Geometry: final body of the model. Coordinates: model frame, mm. Face numbers are marked on the shaded views. A direction names the side the tool comes from. Give positions to 0.01 mm unless a question says otherwise; leave off trailing zeros. Write each loop counter-clockwise with the first axis right and the second up, starting at its lowest first coordinate (ties: lowest second). Pieces come first, ordered by that corner, then holes.
```python
from build123d import *

# Parameters (mm, degrees)
SKETCH_1_W           = 112
SKETCH_1_H           = 110
EXTRUDE_1_DEPTH      = 126
FILLET_1_R           = 55
SKETCH_9_R           = 42.5
CUT_EXTRUDE_5_DEPTH  = 104
SKETCH_10_R          = 42.5
CUT_EXTRUDE_6_DEPTH  = 57
CUT_EXTRUDE_START    = -50
SKETCH_11_R          = 42.5
CUT_EXTRUDE_7_DEPTH  = 50
CHAMFER_1_SIZE       = 55
CHAMFER_1_SIZE2      = 5
CHAMFER_2_SIZE       = 5
CHAMFER_2_SIZE2      = 55
SKETCH_14_W          = 143.089430894
SKETCH_14_H          = 9
CUT_EXTRUDE_8_DEPTH  = 202.295802241
CHAMFER_5_SIZE       = 4
CHAMFER_6_SIZE       = 4
SKETCH_18_R          = 5
CUT_EXTRUDE_9_DEPTH  = 21
SKETCH_19_R          = 45
CUT_EXTRUDE_10_DEPTH = 11
CUT_EXTRUDE_START_2  = -11
SKETCH_20_R          = 45
CUT_EXTRUDE_11_DEPTH = 11
CHAMFER_7_SIZE       = 4
SKETCH_17_R          = 47.5
SKETCH_17_R_2        = 42.5
CUT_EXTRUDE_12_DEPTH = 2
CHAMFER_8_SIZE       = 1
SKETCH_21_R          = 5
CUT_EXTRUDE_13_DEPTH = 10
SKETCH_22_R          = 2
CUT_EXTRUDE_14_DEPTH = 10


# Some blends are built 0.0001 mm under size
with BuildPart() as part:
    # 草图1 → 拉伸1 (new body)
    with BuildSketch(Plane.XY):
        with Locations((56, -55)):
            Rectangle(SKETCH_1_W, SKETCH_1_H)
    extrude(amount=EXTRUDE_1_DEPTH)

    # 圆角1
    fillet_1_edges = [part.edges().sort_by_distance(p)[0] for p in [
        (112, -110, 63),
        (112, 0, 63),
    ]]
    fillet(fillet_1_edges, radius=FILLET_1_R - 0.0001)  # a hair under: the kernel refuses the full size

    # 草图9 → 切除-拉伸5 (cut)
    with BuildSketch(Plane.XY.offset(126)):
        with Locations((57, -55)):
            Circle(SKETCH_9_R)
    extrude(amount=-CUT_EXTRUDE_5_DEPTH, mode=Mode.SUBTRACT)

    # 草图10 → 切除-拉伸6 (cut)
    with BuildSketch(Plane.ZY):
        with Locations(Location((63, -55, 0), (0, 0, 270))):
            Circle(SKETCH_10_R)
    extrude(amount=-CUT_EXTRUDE_6_DEPTH, mode=Mode.SUBTRACT)

    # 草图11 → 切除-拉伸7 (cut)
    with BuildSketch(Plane(origin=(0, 0, 0), x_dir=(-1, 0, 0), z_dir=(0, 0, -1)).offset(CUT_EXTRUDE_START)):
        with Locations(Location((-57, -55, 0), (0, 0, 180))):
            Circle(SKETCH_11_R)
    extrude(amount=CUT_EXTRUDE_7_DEPTH, mode=Mode.SUBTRACT)

    # 倒角1
    chamfer_1_edges = [part.edges().sort_by_distance(p)[0] for p in [
        (0, 0, 63),
    ]]
    chamfer_1_side = [part.faces().sort_by_distance(p)[0] for p in [
        (28.50005, 0, 63),
    ]]
    chamfer(chamfer_1_edges, length=CHAMFER_1_SIZE, length2=CHAMFER_1_SIZE2, reference=chamfer_1_side[0])

    # 倒角2
    chamfer_2_edges = [part.edges().sort_by_distance(p)[0] for p in [
        (0, -110, 63),
    ]]
    chamfer_2_side = [part.faces().sort_by_distance(p)[0] for p in [
        (0, -57.5, 1.640152432),
    ]]
    chamfer(chamfer_2_edges, length=CHAMFER_2_SIZE, length2=CHAMFER_2_SIZE2, reference=chamfer_2_side[0])

    # 草图14 → 切除-拉伸8 (cut, through all)
    with BuildSketch(Plane(origin=(0, 0, 0), x_dir=(1, 0, 0), z_dir=(0, 1, 0))):
        with Locations((58.317073171, -4.5)):
            Rectangle(SKETCH_14_W, SKETCH_14_H)
        with Locations((58.317073171, -121.5)):
            Rectangle(SKETCH_14_W, SKETCH_14_H)
    extrude(amount=-CUT_EXTRUDE_8_DEPTH, mode=Mode.SUBTRACT)

    # 倒角5
    chamfer_5_edges = [part.edges().sort_by_distance(p)[0] for p in [
        (0, -55, 117),
    ]]
    chamfer(chamfer_5_edges, length=CHAMFER_5_SIZE)

    # 倒角6
    chamfer_6_edges = [part.edges().sort_by_distance(p)[0] for p in [
        (0, -55, 9),
    ]]
    chamfer(chamfer_6_edges, length=CHAMFER_6_SIZE)

    # 草图18 → 切除-拉伸9 (cut)
    with BuildSketch(Plane.ZY):
        with Locations((23, -15)):
            Circle(SKETCH_18_R)
        with Locations((103, -15)):
            Circle(SKETCH_18_R)
        with Locations((23, -95)):
            Circle(SKETCH_18_R)
        with Locations((103, -95)):
            Circle(SKETCH_18_R)
    extrude(amount=-CUT_EXTRUDE_9_DEPTH, mode=Mode.SUBTRACT)

    # 草图19 → 切除-拉伸10 (cut)
    with BuildSketch(Plane.XY.offset(117)):
        with Locations((57, -55)):
            Circle(SKETCH_19_R)
    extrude(amount=-CUT_EXTRUDE_10_DEPTH, mode=Mode.SUBTRACT)

    # 草图20 → 切除-拉伸11 (cut)
    with BuildSketch(Plane(origin=(0, 0, 9), x_dir=(-1, 0, 0), z_dir=(0, 0, -1)).offset(CUT_EXTRUDE_START_2)):
        with Locations(Location((-57, -55, 0), (0, 0, 180))):
            Circle(SKETCH_20_R)
    extrude(amount=CUT_EXTRUDE_11_DEPTH, mode=Mode.SUBTRACT)

    # 倒角7
    # the kernel refuses this chamfer: 4 mm, written as the material it takes off along each edge
    with BuildSketch(Plane(origin=(-6.244486468, -104.432319412, 117), x_dir=(-0.002489359702032544, -0.027382956722357982, -0.9996219169112968), z_dir=(0.9958932064677039, -0.09053574604251853, 0)), Plane(origin=(65.244486468, 0.931316952, 117), x_dir=(-0.002489359702032457, 0.027382956722357025, -0.9996219169112968), z_dir=(-0.9958932064677039, -0.09053574604251853, 0))) as chamfer_7_piece_1:
        Polygon((CHAMFER_7_SIZE * 0.999621916911, CHAMFER_7_SIZE * 0.0274958766106), (-CHAMFER_7_SIZE * 0.0274958766106, CHAMFER_7_SIZE * 0.999621916911), (0, 0), align=None)
    extrude(amount=71.783774074, mode=Mode.SUBTRACT)
    with BuildSketch(Plane(origin=(57.0001, -110, 117), x_dir=(0, 0.9996219169112968, 0.027495876610585647), z_dir=(-1, 0, 0)), Plane(origin=(44.713268048, 0, 117), x_dir=(0, -0.9996219169112968, 0.02749587661058563), z_dir=(1, 0, 0))) as chamfer_7_piece_2:
        Polygon((CHAMFER_7_SIZE * 0.999621916911, CHAMFER_7_SIZE * 0.0274958766106), (-CHAMFER_7_SIZE * 0.0274958766106, CHAMFER_7_SIZE * 0.999621916911), (0, 0), align=None)
    extrude(amount=12.286831952, mode=Mode.SUBTRACT)
    with BuildSketch(Plane(origin=(57.0001, -55.0001, 117), x_dir=(0, -1, 0), z_dir=(-1, 0, 0))) as chamfer_7_piece_3:
        Polygon((54.9999 - CHAMFER_7_SIZE, 0), (54.9999, -CHAMFER_7_SIZE), (54.9999, 0), align=None)
    revolve(axis=Axis((57.0001, -55.0001, 117), (0, 0, 1)), revolution_arc=90, mode=Mode.SUBTRACT)
    with BuildSketch(Plane(origin=(57.0001, -54.9999, 117), x_dir=(1, 0, 0), z_dir=(0, -1, 0))) as chamfer_7_piece_4:
        Polygon((54.9999 - CHAMFER_7_SIZE, 0), (54.9999, -CHAMFER_7_SIZE), (54.9999, 0), align=None)
    revolve(axis=Axis((57.0001, -54.9999, 117), (0, 0, 1)), revolution_arc=90, mode=Mode.SUBTRACT)
    with BuildSketch(Plane(origin=(-6.244486468, -104.432319412, 9), x_dir=(-0.002489359702032431, -0.027382956722357972, 0.9996219169112968), z_dir=(0.9958932064677039, -0.09053574604251853, 0)), Plane(origin=(65.244486468, 0.931316952, 9), x_dir=(-0.0024893597020323437, 0.02738295672235701, 0.9996219169112968), z_dir=(-0.9958932064677039, -0.09053574604251853, 0))) as chamfer_7_piece_5:
        Polygon((CHAMFER_7_SIZE * 0.999621916911, -CHAMFER_7_SIZE * 0.0274958766106), (-CHAMFER_7_SIZE * 0.0274958766106, -CHAMFER_7_SIZE * 0.999621916911), (0, 0), align=None)
    extrude(amount=71.783774074, mode=Mode.SUBTRACT)
    with BuildSketch(Plane(origin=(44.713268048, 0, 9), x_dir=(0, -0.9996219169112968, -0.027495876610586494), z_dir=(1, 0, 0)), Plane(origin=(57.0001, -110, 9), x_dir=(0, 0.9996219169112968, -0.02749587661058651), z_dir=(-1, 0, 0))) as chamfer_7_piece_6:
        Polygon((CHAMFER_7_SIZE * 0.999621916911, -CHAMFER_7_SIZE * 0.0274958766106), (-CHAMFER_7_SIZE * 0.0274958766106, -CHAMFER_7_SIZE * 0.999621916911), (0, 0), align=None)
    extrude(amount=12.286831952, mode=Mode.SUBTRACT)
    with BuildSketch(Plane(origin=(57.0001, -54.9999, 9), x_dir=(1, 0, 0), z_dir=(0, -1, 0))) as chamfer_7_piece_7:
        Polygon((54.9999 - CHAMFER_7_SIZE, 0), (54.9999, CHAMFER_7_SIZE), (54.9999, 0), align=None)
    revolve(axis=Axis((57.0001, -54.9999, 9), (0, 0, 1)), revolution_arc=90, mode=Mode.SUBTRACT)
    with BuildSketch(Plane(origin=(57.0001, -55.0001, 9), x_dir=(0, -1, 0), z_dir=(-1, 0, 0))) as chamfer_7_piece_8:
        Polygon((54.9999 - CHAMFER_7_SIZE, 0), (54.9999, CHAMFER_7_SIZE), (54.9999, 0), align=None)
    revolve(axis=Axis((57.0001, -55.0001, 9), (0, 0, 1)), revolution_arc=90, mode=Mode.SUBTRACT)
    with BuildSketch(Plane(origin=(112, -54.9999, 9), x_dir=(-0.9996219169112968, 0, -0.02749587661058651), z_dir=(0, -1, 0))) as chamfer_7_piece_9:
        Polygon((CHAMFER_7_SIZE * 0.999621916911, -CHAMFER_7_SIZE * 0.0274958766106), (-CHAMFER_7_SIZE * 0.0274958766106, -CHAMFER_7_SIZE * 0.999621916911), (0, 0), align=None)
    extrude(amount=0.0002, mode=Mode.SUBTRACT)
    with BuildSketch(Plane(origin=(112, -54.9999, 117), x_dir=(-0.9996219169112968, 0, 0.027495876610585647), z_dir=(0, -1, 0))) as chamfer_7_piece_10:
        Polygon((CHAMFER_7_SIZE * 0.999621916911, CHAMFER_7_SIZE * 0.0274958766106), (-CHAMFER_7_SIZE * 0.0274958766106, CHAMFER_7_SIZE * 0.999621916911), (0, 0), align=None)
    extrude(amount=0.0002, mode=Mode.SUBTRACT)

    # 草图17 → 切除-拉伸12 (cut)
    with BuildSketch(Plane.ZY):
        with Locations(Location((63, -55, 0), (0, 0, 270))):
            Circle(SKETCH_17_R)
        with Locations(Location((63, -55, 0), (0, 0, 270))):
            Circle(SKETCH_17_R_2, mode=Mode.SUBTRACT)
    extrude(amount=-CUT_EXTRUDE_12_DEPTH, mode=Mode.SUBTRACT)

    # 倒角8
    chamfer_8_edges = [part.edges().sort_by_distance(p)[0] for p in [
        (2, -12.5, 63),
    ]]
    chamfer(chamfer_8_edges, length=CHAMFER_8_SIZE)

    # 草图21 → 切除-拉伸13 (cut)
    with BuildSketch(Plane.XZ.offset(110)):
        with Locations(Location((57, 98, 0), (0, 0, 270))):
            Circle(SKETCH_21_R)
        with Locations(Location((57, 78, 0), (0, 0, 90))):
            Circle(SKETCH_21_R)
    extrude(amount=-CUT_EXTRUDE_13_DEPTH, mode=Mode.SUBTRACT)

    # 草图22 → 切除-拉伸14 (cut)
    with BuildSketch(Plane.XZ.offset(100)):
        with Locations(Location((57, 78, 0), (0, 0, 270))):
            Circle(SKETCH_22_R)
        with Locations(Location((57, 98, 0), (0, 0, 270))):
            Circle(SKETCH_22_R)
    extrude(amount=-CUT_EXTRUDE_14_DEPTH, mode=Mode.SUBTRACT)


solid = part.part
```
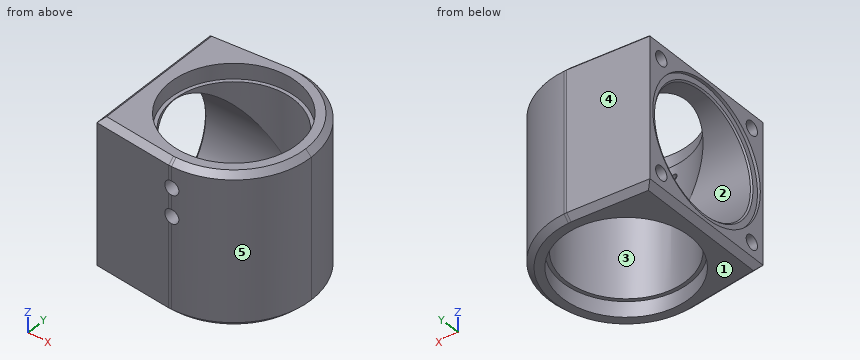
Item 1: Pin query (flat end, axial travel): pin 1 Ø8 at (y, z) = (-95, 23) entering from +X; pin 2 Ø4 at (x, y) = (49, -95.5) entering from -Z; pin 3 Ø4 at (y, z) = (-15.5, 87) entering from +X; pin 4 Ø16 at (y, z) = (-95, 103) entering from -X. Return the tip coordinate at first contact, or that it passes through.
Found:
pin 1: stops at x = 98.58
pin 2: stops at z = 20
pin 3: stops at x = 97.23
pin 4: stops at x = 0
Item 2: Line query: L1, parallel to X at y = -55, z = 77; L2, parallel to X at y = -98.4, z = 98; L3, parallel to Y at x = 57, z = 12.75. Output: solid intervals per line, ascending.
Found:
L1: x = 99.5 to 112
L2: x = 0 to 55, 59 to 90.79
L3: y = -109.75 to -100, -10 to -0.25
Item 3: Pull-direction query (X, two-part tool) for the marked faces 3, 4 and 5; classes: +X half, -X half, draft (parallel to the pull), parting line (faces both ways), or undercut.
Found:
face 3: undercut
face 4: -X half
face 5: +X half
Item 4: Section C-C, the plane y = -35. State how many separate pieces and enclosed holes the cut face has, plus the area to 3 significant figures.
Found:
separate pieces: 3
enclosed holes: 0
area: 1,950 mm2
Item 5: Reachability of the marked faces 1 and 2 from +Z, -Z, +X, -X, +Y, -Y: full face, straight path, thin tool, end or side. Return the list, or none.
Found:
face 1: -Z, +X, -X, +Y, -Y
face 2: -X
Item 6: Section A-A, the plane x = 48. Return the cut outline in (y, z), plus the area to 3 significant figures.
Found:
outline: (-109.36, 13) - (-105.35, 9) - (-99.09, 9) - (-99.09, 20) - (-96.54, 20) - (-96.54, 54) arc R42.5 cw to (-96.54, 72) - (-96.54, 106) - (-99.09, 106) - (-99.09, 117) - (-105.35, 117) - (-109.36, 113) - close; (-13.46, 20) - (-10.91, 20) - (-10.91, 9) - (-4.65, 9) - (-0.64, 13) - (-0.64, 113) - (-4.65, 117) - (-10.91, 117) - (-10.91, 106) - (-13.46, 106) - (-13.46, 72) arc R42.5 cw to (-13.46, 54) - close
area: 2,600 mm2
